Could you check a few things on this model? Use its own coordinates, in mm. A direction names the side the tool comes from. Coordinates: 2 decimals unless noted, no trailing zeros. Order: outer loops, then holes, each group sorted by start corner. A loop starts at its lowest first (then second) coordinate and runs counter-clockwise, first axis right, second up. Notation, with made-up numbers: (-29.5, -5.75) -> (-5.5, -5.75) arc R17 ccw to (-5.5, 6.25) -> close; hole circle Ø1 at (-37.5, 10.25). An arc over 180 degrees is marked (long way). Put each result on its own line as item: value. Start each with the question number.
Q1. If we section it at C-C (y = -19.5): Please give me the cut outline in (x, z), and give its area (3 significant figures).
Q2. If we section it at D-D (y = -5.5): Please give me the cut outline in (x, z), and give its area (3 significant figures).
Q3. For faces 1 (the face through (56, -19, 2)), 2 (the face through (-14, -12, 2)), which set-ups out of +Z, -Z, +X, -X, +Y, -Y let a thin tool reach every point of the face, with its end or its side?
Q4. If we section it at B-B (z = 3.4): Please give me the cut outline in (x, y).
Q5. If we section it at A-A (x = 33): Please give me the cut outline in (y, z).
Q6. Will these pins go through, and if not, where does the flat tip stop? pin 1 (2 mm diameter, centred on x = -2.5, z = 1.5, fed in from -Y); pin 2 (8 mm diameter, centred on x = 26, y = -12.5, fed in from -Z).
Q7. Please list where these lines run through material, in increasing order: line 1 along X through (y, z) = (-19.5, 1.55); line 2 along Y through (x, z) = (26, 1.5); line 3 along X through (y, z) = (-23.25, 3.2).
Q8. We'd pull the mould along X, two halves only. Please class faces 3 (the face through (-4, -19, 2)), 4 (the face through (25, -18, 4)), 5 (the face through (65.43, -0.6, 2.03)): +X half, -X half, draft (parallel to the pull), parting line (faces both ways), or undercut.
Autodesk Inventor part; units mm, degrees
ref_plane "YZ Plane" through (0, 0, 0) normal (1, 0, 0) x (0, 1, 0)
ref_plane "XZ Plane" through (0, 0, 0) normal (0, 1, 0) x (-1, 0, 0)
ref_plane "XY Plane" through (0, 0, 0) normal (0, 0, 1) x (1, 0, 0)
sketch "Эскиз1" plane through (0, 0, 0) normal (0, 0, 1) x (1, 0, 0)
  line L0 (0, 0) -> (52, 0)
  line L1 (52, 0) -> (52, -25)
  line L2 (52, -25) -> (0, -25)
  line L3 (0, -25) -> (0, 0)
  line L4 (0, -12.5) -> (-4, -12.5)
  line L5 (-4, -12.5) -> (-4, 0)
  line L6 (-4, 0) -> (0, 0)
  line L7 (0, 0) -> (0, -12.5)
  line L8 (-4, 0) -> (-14, 0)
  line L9 (-14, 0) -> (-14, -25)
  line L10 (-14, -25) -> (-4, -25)
  line L11 (-4, -25) -> (-4, 0)
  line L12 (52, -12.5) -> (56, -12.5)
  line L13 (56, -12.5) -> (56, 0)
  line L14 (56, 0) -> (52, 0)
  line L15 (52, 0) -> (52, -12.5)
  line L16 (56, 0) -> (66, 0)
  line L17 (66, 0) -> (66, -25)
  line L18 (66, -25) -> (56, -25)
  line L19 (56, -25) -> (56, 0)
  circle A0 centre (26, -12.5) radius 3
  circle A1 centre (26, -12.5) radius 7
  circle A2 centre (33, -12.5) radius 1.5
  circle A3 centre (19, -12.5) radius 1.5
  circle A4 centre (26, -5.5) radius 1.5
  circle A5 centre (26, -19.5) radius 1.5
  dimension "d0" = 52
  dimension "d1" = 25
  dimension "d2" = 4
  dimension "d3" = 10
  dimension "d4" = 4
  dimension "d5" = 10
  dimension "d9" = 6
  dimension "d10" = 14
  dimension "d11" = 3
  dimension "d12" = 3
  dimension "d13" = 3
  dimension "d14" = 3
extrude "Выдавливание1" add sketch "Эскиз1" along normal blind 4 contours L0 L1 L2 L3 | L3 L4 L5 L6 | L14 L13 L12 L1 | L5 L11 L10 L9 L8 | L16 L17 L18 L19 L13 | A2 A1 A5 A3 A4
fillet "Сопряжение1" radius 2 4 edges at (66, 0, 2) (66, -25, 2) (-14, -25, 2) (-14, 0, 2)
properties material "Дерево (вишня)"
The answers:
1. outline: (-14, 0) -> (-4, 0) -> (-4, 4) -> (-14, 4) -> close; (0, 0) -> (24.5, 0) -> (24.5, 4) -> (0, 4) -> close; (27.5, 0) -> (52, 0) -> (52, 4) -> (27.5, 4) -> close; (56, 0) -> (66, 0) -> (66, 4) -> (56, 4) -> close
1. area: 276 mm^2
2. outline: (-14, 0) -> (24.5, 0) -> (24.5, 4) -> (-14, 4) -> close; (27.5, 0) -> (66, 0) -> (66, 4) -> (27.5, 4) -> close
2. area: 308 mm^2
3. face 1: +Z, -Z, -Y
3. face 2: +Z, -Z, -X, +Y, -Y
4. outline: (-14, -23) arc R2 ccw to (-12, -25) -> (-4, -25) -> (-4, -12.5) -> (0, -12.5) -> (0, -25) -> (52, -25) -> (52, -12.5) -> (56, -12.5) -> (56, -25) -> (64, -25) arc R2 ccw to (66, -23) -> (66, -2) arc R2 ccw to (64, 0) -> (-12, 0) arc R2 ccw to (-14, -2) -> close; hole circle Ø3 at (19, -12.5); hole circle Ø6 at (26, -12.5); hole circle Ø3 at (26, -19.5); hole circle Ø3 at (26, -5.5); hole circle Ø3 at (33, -12.5)
5. outline: (-25, 0) -> (-14, 0) -> (-14, 4) -> (-25, 4) -> close; (-11, 0) -> (0, 0) -> (0, 4) -> (-11, 4) -> close
6. pin 1: y = -12.5
6. pin 2: z = 0
7. line 1: -14 to -4, 0 to 24.5, 27.5 to 52, 56 to 66
7. line 2: -25 to -21, -18 to -15.5, -9.5 to -7, -4 to 0
7. line 3: -13.98 to -4, 0 to 52, 56 to 65.98
8. face 3: undercut
8. face 4: draft
8. face 5: +X half
